Verification items for this drawing (mm, ordinates from the low corner). Give positions to 0.01 mm unless a question says otherwise; leave off trailing zeros. Loops run counter-clockwise (first coordinate to the right, second up) from the corner with the lowest first, then second, coordinate; pieces in that order, holes last. Notation, with made-up numbers: M -38.75,70 L -25.75,70 A17 ccw -25.75,102 Z; hole C 57,23 d10. An arc over 180 degrees is marked long. Use a Markdown table: item, result.
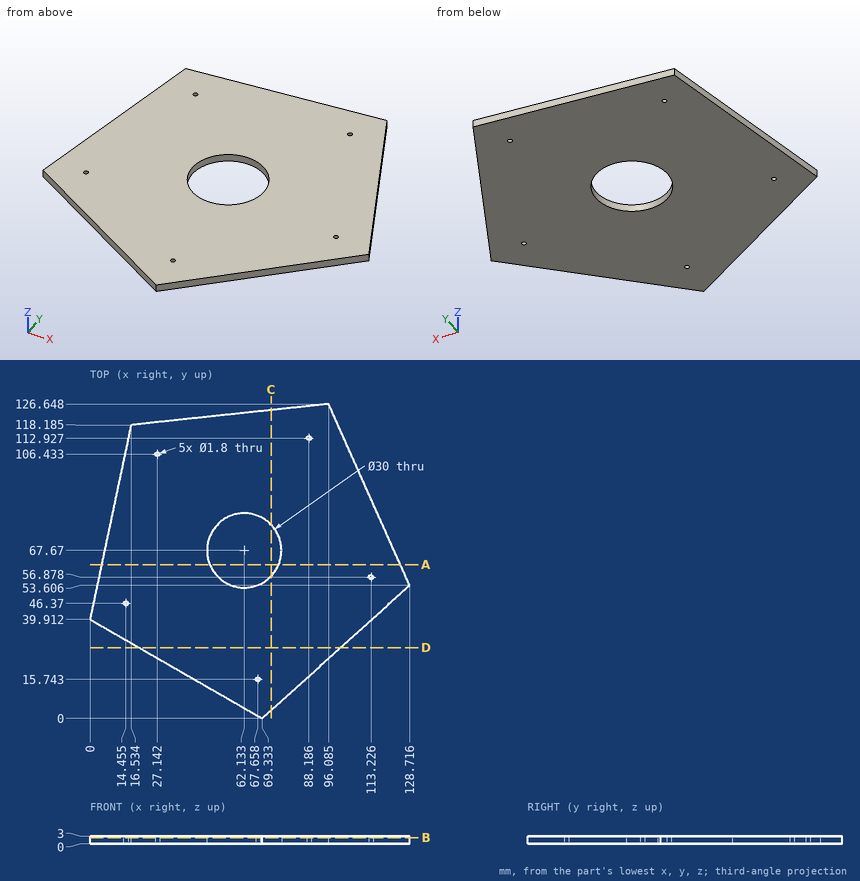
(1) Cross-section at B-B on z = 2.5. Record the cut outline in (x, y) (1 decimal), then the cut area to 3 significant figures.
Results below:
| item | result |
|---|---|
| outline | M 0,39.9 L 69.3,0 L 128.7,53.6 L 96.1,126.6 L 16.5,118.2 Z; hole C 14.5,46.4 d1.8; hole C 27.1,106.4 d1.8; hole C 62.1,67.7 d30; hole C 67.7,15.7 d1.8; hole C 88.2,112.9 d1.8; hole C 113.2,56.9 d1.8 |
| area | 10,300 mm^2 |
(2) Gauge pin test, flat end, axial feed: P1, Ø1, axis at y = 88, z = 1.5, coming from the +X side (1 decimal). Record the tip position at first contact, or that the pin passes through.
Results below:
| item | result |
|---|---|
| P1 | x = 113.6 |
(3) Material ranges on line 1 (Y direction, x = 53, z = 2.7) (1 decimal); line 2 (Y direction, x = 87.5, z = 1.35) (1 decimal); line 3 (X direction, y = 58.5, z = 1.7) (1 decimal), recorded low to high.
Results below:
| item | result |
|---|---|
| line 1 | 9.4 to 55.8, 79.6 to 122.1 |
| line 2 | 16.4 to 112.3, 113.5 to 125.7 |
| line 3 | 3.9 to 50.3, 74 to 126.5 |
(4) Cross-section at D-D on y = 28.5. Record the cut outline in (x, z) (1 decimal).
Results below:
| item | result |
|---|---|
| outline | M 19.8,0 L 100.9,0 L 100.9,3 L 19.8,3 Z |
(5) Cross-section at C-C on x = 73. Record the cut outline in (y, z).
Results below:
| item | result |
|---|---|
| outline | M 3.31,0 L 57.33,0 L 57.33,3 L 3.31,3 Z; M 78.01,0 L 124.19,0 L 124.19,3 L 78.01,3 Z |
(6) Cross-section at A-A on y = 62. Record the cut outline in (x, z) (1 decimal).
Results below:
| item | result |
|---|---|
| outline | M 4.7,0 L 48.2,0 L 48.2,3 L 4.7,3 Z; M 76,0 L 125,0 L 125,3 L 76,3 Z |
